Could you check a few things on this model? Use its own coordinates, in mm. Round coordinates to 2 decimals unless told otherwise and drop trailing zeros. Loops run counter-clockwise (first coordinate to the right, second up) from the corner with the lowest first, then second, coordinate; pieces in that order, holes last. Notation, with made-up numbers: (1.25, -23.5) - (31.25, -23.5) arc R23 ccw to (31.25, 4.5) - close; hole circle Ø6 at (-27, 55). An arc over 180 degrees is marked (long way). Put each result on its own line as item: value. Start each with the question number.
from build123d import *

# Parameters (mm, degrees)
F0_W     = 40
F0_H     = 15
F1_DEPTH = 5
F2_R     = 5
F3_R     = 5


with BuildPart() as f1:
    # F0 (on Top) → F1 (new body)
    with BuildSketch(Plane.XY):
        with Locations((20, -7.5)):
            Rectangle(F0_W, F0_H)
    extrude(amount=F1_DEPTH)

    # F2
    f2_edges = [f1.edges().sort_by_distance(p)[0] for p in [
        (40, -15, 2.5),
        (40, 0, 2.5),
    ]]
    fillet(f2_edges, radius=F2_R)

    # F3
    f3_edges = [f1.edges().sort_by_distance(p)[0] for p in [
        (0, -15, 2.5),
        (0, 0, 2.5),
    ]]
    fillet(f3_edges, radius=F3_R)


solid = f1.part
Item 1: I need wall thicknesses on line 1 (X direction, y = -12, z = 1.55); line 2 (X direction, y = -1.5, z = 2.2); line 3 (Y direction, x = 36.5, z = 4.2). Which ranges of each line are inside material? Lowest first, please. Write a range as from..to.
Item 2: Suppose I cut it at A-A, the plane z = 3.65. List the corners of the cut face in (x, y) for me.
Item 3: Suppose I cut it at B-B, the plane y = -11.75. List the corners of the cut face in (x, z) for me, then the cut area to 3 significant figures.
Numbers:
1. line 1: 0.42..39.58
1. line 2: 1.43..38.57
1. line 3: -14.77..-0.23
2. outline: (0, -10) arc R5 ccw to (5, -15) - (35, -15) arc R5 ccw to (40, -10) - (40, -5) arc R5 ccw to (35, 0) - (5, 0) arc R5 ccw to (0, -5) - close
3. outline: (0.32, 0) - (39.68, 0) - (39.68, 5) - (0.32, 5) - close
3. area: 197 mm^2
